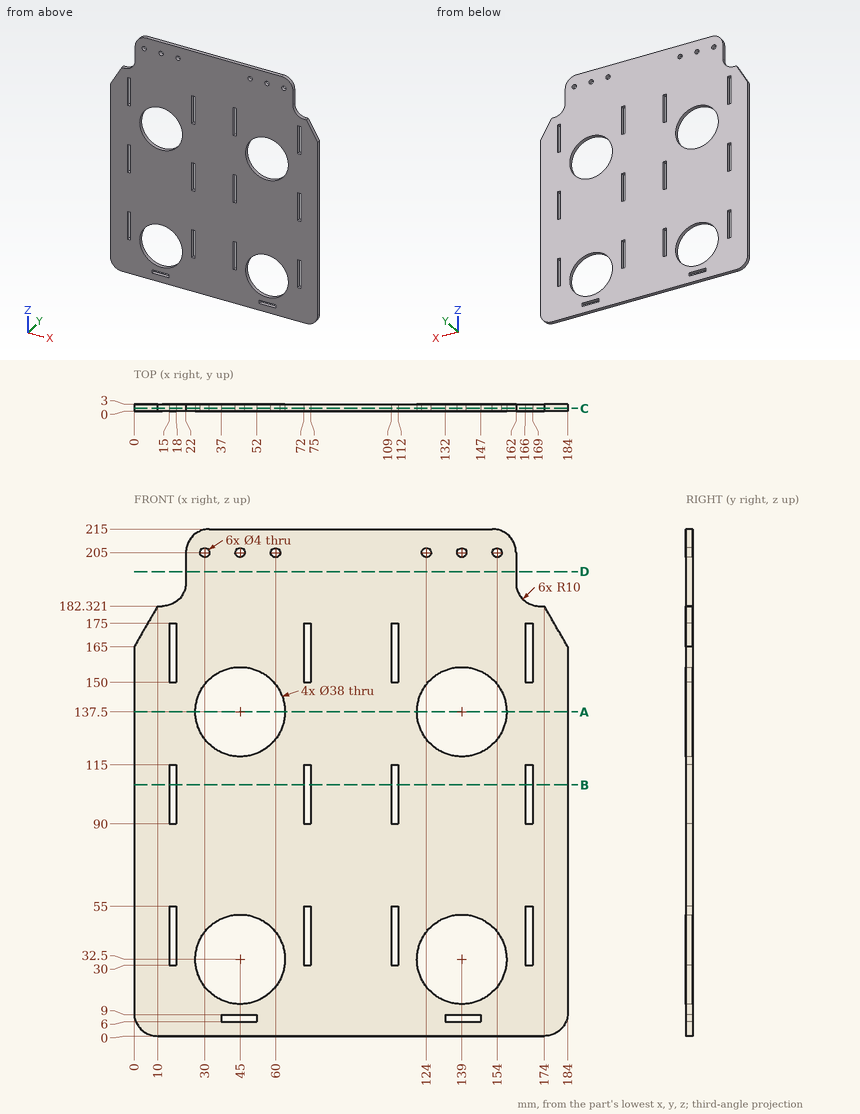
Could you check a few things on this drawing? It's one solid part, dimensions in mm from its lowest x, y, z. Coordinates: 2 decimals unless noted, no trailing zeros. Order: outer loops, then holes, each group sorted by start corner. A loop starts at its lowest first (then second) coordinate and runs counter-clockwise, first axis right, second up. Notation, with made-up numbers: M 33,11 L 75,11 A17 ccw 75,16 Z; hole C 10,57 d8. An arc over 180 degrees is marked long. Use a Markdown table: item, result. Add a question column.
Q1. If I drill on L1, parallel to X at y = 0.6, z = 137.5; L2, parallel to Z at x = 16, y = 2.8 (1 decimal); L3, parallel to Z at x = 29.5, y = 1 (1 decimal), over which ranges is the centre line in solid material (lowest first)?
Q2. I want a section at C-C on y = 1.1. Give the number of separate pieces and of enclosed holes in the cut face, then the cut area to 3 significant figures.
Q3. I want a section at A-A on z = 137.5. List the corners of the cut face in (x, y) for me, then the cut area to 3 significant figures.
Q4. I'm going to push flat-ended pins straight in: pin 1 (1.5 mm diameter, centred on y = 1, z = 169, fed in from +X); pin 2 (1.6 mm diameter, centred on x = 11.5, y = 1.5, fed in from +Z) (1 decimal). Where does each tip first touch, or does it pass through?
Q5. I want a section at B-B on z = 106.5. List the corners of the cut face in (x, y) for me.
Q6. I want a section at D-D on z = 197. List the corners of the cut face in (x, y) for me, then the cut area to 3 significant figures.
Checked values:
| question | item | result |
|---|---|---|
| 1 | L1 | 0 to 26, 64 to 120, 158 to 184 |
| 1 | L2 | 0 to 30, 55 to 90, 115 to 150, 175 to 183.2 |
| 1 | L3 | 0 to 21.5, 43.5 to 126.5, 148.5 to 203.1, 206.9 to 214.7 |
| 2 | separate pieces | 1 |
| 2 | enclosed holes | 24 |
| 2 | area | 32,300 mm² |
| 3 | outline | M 0,0 L 26,0 L 26,3 L 0,3 Z; M 64,0 L 120,0 L 120,3 L 64,3 Z; M 158,0 L 184,0 L 184,3 L 158,3 Z |
| 3 | area | 324 mm² |
| 4 | pin 1 | x = 182.12 |
| 4 | pin 2 | z = 182.3 |
| 5 | outline | M 0,0 L 15,0 L 15,3 L 0,3 Z; M 18,0 L 72,0 L 72,3 L 18,3 Z; M 75,0 L 109,0 L 109,3 L 75,3 Z; M 112,0 L 166,0 L 166,3 L 112,3 Z; M 169,0 L 184,0 L 184,3 L 169,3 Z |
| 6 | outline | M 22,0 L 162,0 L 162,3 L 22,3 Z |
| 6 | area | 420 mm² |
